from build123d import *

# Parameters (mm, degrees)
SKETCH1_W              = 184.15
SKETCH1_H              = 50.8
BOSS_EXTRUDE1_DEPTH    = 9.525
SKETCH4_W              = 88.9
SKETCH4_H              = 6.35
BOSS_EXTRUDE2_DEPTH    = 50.8
SKETCH5_W              = 57.15
SKETCH5_H              = 50.8
CUT_EXTRUDE1_DEPTH     = 9.525
F_10_CLEARANCE_HOLE1_D = 5.1054
FILLET1_R              = 3.175
CHAMFER1_SIZE          = 3.175


# Some blends are built 0.0001 mm under size
with BuildPart() as part:
    # Sketch1 → Boss-Extrude1 (new body)
    with BuildSketch(Plane(origin=(0, 0, 0), x_dir=(1, 0, 0), z_dir=(0, 1, 0))):
        with Locations((92.075, 25.4)):
            Rectangle(SKETCH1_W, SKETCH1_H)
    extrude(amount=BOSS_EXTRUDE1_DEPTH)

    # Sketch4 → Boss-Extrude2 (add)
    with BuildSketch(Plane.XY):
        with Locations((92.075, -3.175)):
            Rectangle(SKETCH4_W, SKETCH4_H)
    extrude(amount=-BOSS_EXTRUDE2_DEPTH)

    # Sketch5 → Cut-Extrude1 (cut)
    with BuildSketch(Plane(origin=(0, 9.525, 0), x_dir=(1, 0, 0), z_dir=(0, 1, 0))):
        with Locations((92.075, 25.4)):
            Rectangle(SKETCH5_W, SKETCH5_H)
    extrude(amount=-CUT_EXTRUDE1_DEPTH, mode=Mode.SUBTRACT)

    # #10 Clearance Hole1 (through all)
    with Locations(Plane(origin=(0, 9.525, 0), x_dir=(1, 0, 0), z_dir=(0, 1, 0))):
        with Locations((9.525, 38.1), (9.525, 12.7), (60.325, 12.7), (60.325, 38.1), (123.825, 38.1), (123.825, 12.7), (174.625, 12.7), (174.625, 38.1)):
            Hole(F_10_CLEARANCE_HOLE1_D / 2)

    # Fillet1
    fillet1_edges = [part.edges().sort_by_distance(p)[0] for p in [
        (47.625, 0, -25.4),
        (47.625, -6.35, -25.4),
        (136.525, -6.35, -25.4),
        (63.5, 0, -25.4),
        (120.65, 0, -25.4),
    ]]
    fillet(fillet1_edges, radius=FILLET1_R - 0.0001)  # a hair under: the kernel refuses the full size

    # Chamfer1
    # the kernel refuses this chamfer: 3.175 mm, written as the material it takes off along each edge
    with BuildSketch(Plane(origin=(141.515193487, -6.35, 0), x_dir=(0, 0.9996219169112966, 0.02749587661058637), z_dir=(-1, 0, 0))) as chamfer1_piece_1:
        Polygon((CHAMFER1_SIZE * 0.999621916911, CHAMFER1_SIZE * 0.0274958766106), (-CHAMFER1_SIZE * 0.0274958766106, CHAMFER1_SIZE * 0.999621916911), (0, 0), align=None)
    extrude(amount=98.880386974, mode=Mode.SUBTRACT)


solid = part.part
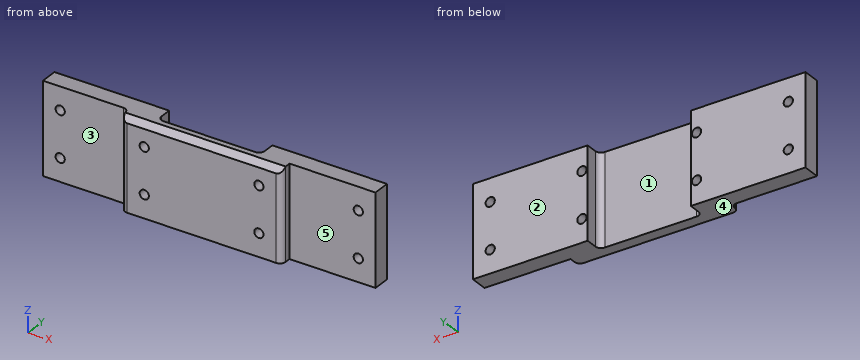
Could you check a few things on this model? Use its own coordinates, in mm. Face numbers are marked on the shaded views. A direction names the side the tool comes from. Give positions to 0.01 mm unless a question says otherwise; leave off trailing zeros. Order: outer loops, then holes, each group sorted by start corner. A loop starts at its lowest first (then second) coordinate and runs counter-clockwise, first axis right, second up. Notation, with made-up numbers: M 50.25,82 L 95.25,82 A14 cw 95.25,88 Z; hole C 31,46.5 d11. An arc over 180 degrees is marked long. One line per question, with ' | ' between items.
1. If I drill on line 1 (X direction, y = -3.25, z = -13); line 2 (X direction, y = 7, z = -12.7); line 3 (X direction, y = 8.25, z = -23.5), over which ranges is the centre line in solid material (lowest first)?
Results:
line 1: 47.63 to 57.79, 62.86 to 121.29, 126.36 to 136.52 | line 2: 0 to 6.97, 12.08 to 57.77, 62.88 to 63.5, 120.65 to 121.27, 126.38 to 172.07, 177.18 to 184.15 | line 3: 0 to 63.5, 120.65 to 184.15
2. For the marked faces 3, 4 and 5, which set-ups out of +Z, -Z, +X, -X, +Y, -Y let a thin tool reach every point of the face, with its end or its side?
Results:
face 3: +Z, -Z, -X, -Y | face 4: -Z, +X, -X, +Y, -Y | face 5: +Z, -Z, +X, -Y
3. I want a section at D-D (x = 61). List the corners of the cut face in (y, z) for me (3 decimals), and give its area (3 significant figures).
Results:
outline: M -6.35,-50.8 L 9.525,-50.8 L 9.525,-40.562 L -6.35,-40.562 Z; M -6.35,-35.638 L 9.525,-35.638 L 9.525,-15.162 L -6.35,-15.162 Z; M -6.35,-10.238 L 9.525,-10.238 L 9.525,0 L -3.175,0 L -6.35,-3.175 Z | area: 645 mm²
4. I'm going to push flat-ended pins straight in: pin 1 (1 mm diameter, centred on x = 159, z = -31, fed in from -Y); pin 2 (5 mm diameter, centred on x = 82.5, z = -8.5, fed in from +Y). Where does each tip first touch, or does it pass through?
Results:
pin 1: y = 0 | pin 2: y = 0
5. I want a section at C-C (x = 84). List the corners of the cut face in (y, z) for me (3 decimals), and give its area (3 significant figures).
Results:
outline: M -6.35,-50.8 L 0,-50.8 L 0,0 L -3.175,0 L -6.35,-3.175 Z | area: 318 mm²
6. We'd pull the mould along X, two halves only. Please class the marked faces 1 and 2: +X half, -X half, draft (parallel to the pull), parting line (faces both ways), or undercut.
Results:
face 1: undercut | face 2: draft
7. I want a section at A-A (y = 6.5). Give the number of separate pieces and of enclosed holes in the cut face, and give its area (3 significant figures).
Results:
separate pieces: 2 | enclosed holes: 8 | area: 6,290 mm²
